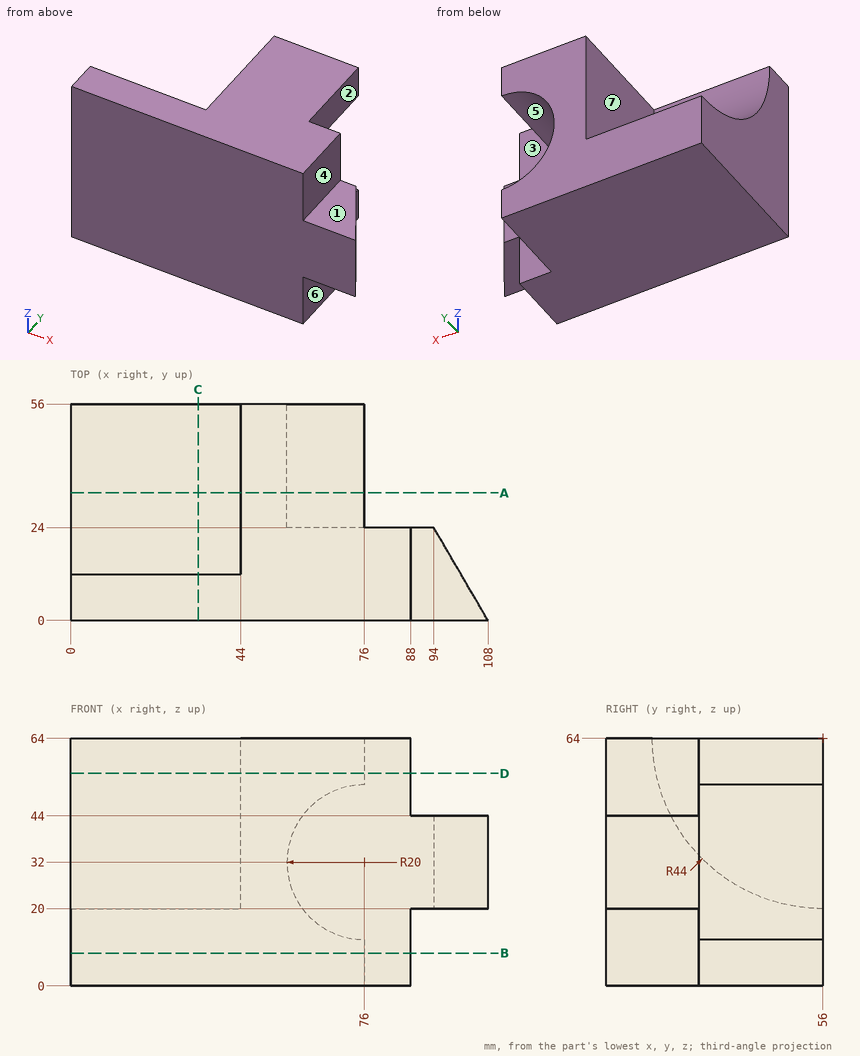
Geometry: see drawing. Coordinates: mm, zero at the bounding-box minimum. A direction names the side the tool comes from. Round coordinates to 2 decimals unless told otherwise and drop trailing zeros. Loops run counter-clockwise (first coordinate to the right, second up) from the corner with the lowest first, then second, coordinate; pieces in that order, holes last. Notation, with made-up numbers: M 51.5,76.5 L 76.5,76.5 A16 ccw 76.5,92.5 Z; hole C -19,73.25 d4. An arc over 180 degrees is marked long. Use a Markdown table: item, result. Add a question column.
1. Contact query for flat-ended pins moving along their axis: P1, Ø3.5, axis at y = 34, z = 6.5, coming from the +X side; P2, Ø10, axis at y = 13.5, z = 36, coming from the +X side; P3, Ø1, axis at x = 18.5, z = 55, coming from the +Y side. Output: stop coordinate, or through.
2. Mould query, pull axis Z, two halves, no side actions, for the marked faces 1, 2 and 3. Classes: pulls with the +Z half, pulls with the -Z half, needs draft (parallel to the pull), parting line crosses it, or undercut.
3. Section query A-A on y = 33. Return the cut outline in (x, z), then the cut area to 3 significant figures.
4. Section query D-D on z = 55. Return the cut outline in (x, y).
5. Section query B-B on z = 8.5. Return the cut outline in (x, y), then the cut area to 3 significant figures.
6. Reachability of the marked faces 4, 5, 6 and 7 from +Z, -Z, +X, -X, +Y, -Y: full face, straight path, thin tool, end or side. Return the list, or none.
7. Section query C-C on x = 33. Return the cut outline in (y, z).
8. Line query: line 1 (X direction, y = 27.5, z = 32.5); line 2 (Z direction, x = 88.5, y = 22); line 3 (Y direction, x = 79.5, z = 41). Output: solid intervals per line, ascending.
Reported:
| question | item | result |
|---|---|---|
| 1 | P1 | stops at x = 76 |
| 1 | P2 | stops at x = 103.04 |
| 1 | P3 | stops at y = 13.04 |
| 2 | face 1 | pulls with the +Z half |
| 2 | face 2 | needs draft |
| 2 | face 3 | undercut |
| 3 | outline | M 0,0 L 76,0 L 76,12 A20 cw 76,52 L 76,64 L 44,64 L 44,26.49 L 0,26.49 Z |
| 3 | area | 2,590 mm² |
| 4 | outline | M 0,0 L 88,0 L 88,24 L 76,24 L 76,56 L 44,56 L 44,12.93 L 0,12.93 Z |
| 5 | outline | M 0,0 L 88,0 L 88,24 L 76,24 L 76,56 L 0,56 Z |
| 5 | area | 4,540 mm² |
| 6 | face 4 | +Z, +X, +Y, -Y |
| 6 | face 5 | +X, +Y |
| 6 | face 6 | -Z, +X, +Y, -Y |
| 6 | face 7 | +Z, -X, +Y |
| 7 | outline | M 0,0 L 56,0 L 56,20 A44 cw 12,64 L 0,64 Z |
| 8 | line 1 | x = 44 to 56.01 |
| 8 | line 2 | z = 20 to 44 |
| 8 | line 3 | y = 0 to 24 |
